from build123d import *

# Parameters (mm, degrees)
SKETCH3_W               = 80
SKETCH3_H               = 40
BOSS_EXTRUDE1_DEPTH     = 20
SKETCH5_R               = 2
CUT_EXTRUDE2_DEPTH      = 40
BOSS_EXTRUDE2_START     = -23
BOSS_EXTRUDE2_OUTLINE_R = 2
BOSS_EXTRUDE2_DEPTH     = 46


# Read off the part's stored shape, not the designer's step: Boss-Extrude2
with BuildPart() as part:
    # Sketch3 → Boss-Extrude1 (new body)
    with BuildSketch(Plane(origin=(0, 0, 0), x_dir=(1, 0, 0), z_dir=(0, 1, 0))):
        Rectangle(SKETCH3_W, SKETCH3_H)
    extrude(amount=BOSS_EXTRUDE1_DEPTH)

    # Sketch5 → Cut-Extrude2 (cut)
    with BuildSketch(Plane.XY.offset(20)):
        with Locations((32.81740635, 10)):
            Circle(SKETCH5_R)
    extrude(amount=-CUT_EXTRUDE2_DEPTH, mode=Mode.SUBTRACT)

    # Boss-Extrude2 outline → Boss-Extrude2 (add)
    with BuildSketch(Plane.XY.offset(BOSS_EXTRUDE2_START)):
        with Locations((32.81740635, 10)):
            Circle(BOSS_EXTRUDE2_OUTLINE_R)
    extrude(amount=BOSS_EXTRUDE2_DEPTH)


solid = part.part
Work out the finished part from the listing and answer in its coordinate system (mm). A direction names the side the tool comes from. Coordinates: 2 decimals unless noted, no trailing zeros. Loops run counter-clockwise (first coordinate to the right, second up) from the corner with the lowest first, then second, coordinate; pieces in that order, holes last. Notation, with made-up numbers: M 59.25,62 L 66.25,62 A8 ccw 66.25,72 Z; hole C 2,19 d9. An arc over 180 degrees is marked long. Answer in a Markdown table with one row per item. Add a question column.
1. Consider L1, parallel to Z at x = 6, y = 14. Determine where the line is inside the solid, lowest interval first.
2. Find section B-B, the plane x = 17.5. Write down the section's boundary in (y, z), then the cut area to 3 significant figures.
3. Find section A-A, the plane y = 10. Write down the section's boundary in (x, z), then the cut area to 3 significant figures.
4. A tool of negligible diameter and unlimited length cuts with its end or side. For faces 1 (the cylindrical face through (31.34, 11.35, 21.48)), 2 (the flat face through (33, 10, -23)), 3 (the cylindrical face through (31.34, 11.35, -21.52)), from which of +Z, -Z, +X, -X, +Y, -Y can it reach the whole face along a straight path? Write none if from no direction.
5. Find section C-C, the plane y = 1.5. Write down the section's boundary in (x, z), then the cut area to 3 significant figures.
6. Flat-ended cylindrical pins translate along their axes: P1, Ø1, axis at x = 12, y = 14, coming from the +Z side; P2, Ø1, axis at x = -4.5, y = 3.5, coming from the -Z side. Find the tip coordinate at first contact, or state that the pin passes through.
Reported:
| question | item | result |
|---|---|---|
| 1 | L1 | z = -20 to 20 |
| 2 | outline | M 0,-20 L 20,-20 L 20,20 L 0,20 Z |
| 2 | area | 800 mm^2 |
| 3 | outline | M -40,-20 L 30.82,-20 L 30.82,-23 L 34.82,-23 L 34.82,-20 L 40,-20 L 40,20 L 34.82,20 L 34.82,23 L 30.82,23 L 30.82,20 L -40,20 Z |
| 3 | area | 3,220 mm^2 |
| 4 | face 1 | +Z |
| 4 | face 2 | -Z, +X, -X, +Y, -Y |
| 4 | face 3 | -Z |
| 5 | outline | M -40,-20 L 40,-20 L 40,20 L -40,20 Z |
| 5 | area | 3,200 mm^2 |
| 6 | P1 | stops at z = 20 |
| 6 | P2 | stops at z = -20 |
